Verification items for the finished model (mm, model axes). Round coordinates to 2 decimals unless told otherwise and drop trailing zeros. Write each loop counter-clockwise with the first axis right and the second up, starting at its lowest first coordinate (ties: lowest second). Pieces come first, ordered by that corner, then holes. Notation, with made-up numbers: M 27.5,67 L 71.5,67 A8 ccw 71.5,73 Z; hole C 86.5,7 d4. An arc over 180 degrees is marked long. One line per item, written item: value. Start each with the question number.
Item 1: Gauge pin test, flat end, axial feed: pin 1 (1.4 mm diameter, centred on x = 52.62, y = 22, fed in from +Z) (3 decimals). Record the tip position at first contact, or that the pin passes through.
Item 2: Thickness scan on probe 1 along Y at (x, z) = (0, 0.45); probe 2 along Y at (x, z) = (-37, 0.25); probe 3 along X at (y, z) = (-24, 0.15). Record the ranges inside material, lowest first. Write a range as from..to.
Item 3: Section check A-A, the plane z = 0.3. Record the cut outline in (x, y).
Item 4: Section check C-C, the plane y = 11. Record the cut outline in (x, z), then the cut area to 3 significant figures.
Item 5: Section check B-B, the plane x = 27. Record the cut outline in (y, z), then the cut area to 3 significant figures.
from build123d import *

# Parameters (mm, degrees)
SKETCH_1_R      = 0.85
EXTRUDE_1_DEPTH = 0.8


with BuildPart() as part:
    # 草图1 → 凸台-拉伸1 (new body)
    with BuildSketch(Plane.XY):
        with BuildLine():
            Line((52.621031394, 26), (-52.621031394, 26))
            ThreePointArc((-52.621031394, 26), (-56.349062871, 23.449752153), (-55.323392225, 19.050890653))
            Line((-55.323392225, 19.050890653), (-2.70236083, -29.167400823))
            ThreePointArc((-2.70236083, -29.167400823), (0, -30.218291475), (2.70236083, -29.167400823))
            Line((2.70236083, -29.167400823), (55.323392225, 19.050890653))
            ThreePointArc((55.323392225, 19.050890653), (56.349062871, 23.449752153), (52.621031394, 26))
        make_face()
        with Locations((-52.621031394, 22)):
            Circle(SKETCH_1_R, mode=Mode.SUBTRACT)
        with Locations((52.621031394, 22)):
            Circle(SKETCH_1_R, mode=Mode.SUBTRACT)
        with Locations((0, -26.218291475)):
            Circle(SKETCH_1_R, mode=Mode.SUBTRACT)
    extrude(amount=EXTRUDE_1_DEPTH)


solid = part.part
Response values:
1. pin 1: passes through
2. probe 1: y = -30.22..-27.07, -25.37..26
2. probe 2: y = 2.26..26
2. probe 3: x = -8.34..8.34
3. outline: M -55.32,19.05 L -2.7,-29.17 A4 ccw 2.7,-29.17 L 55.32,19.05 A4 ccw 52.62,26 L -52.62,26 A4 ccw Z; hole C -52.62,22 d1.7; hole C 0,-26.22 d1.7; hole C 52.62,22 d1.7
4. outline: M -46.54,0 L 46.54,0 L 46.54,0.8 L -46.54,0.8 Z
4. area: 74.5 mm2
5. outline: M -6.9,0 L 26,0 L 26,0.8 L -6.9,0.8 Z
5. area: 26.3 mm2
